Here's how the part is built. I have some questions about the finished solid (model axes, mm). Face numbers are marked on the shaded views. A direction names the side the tool comes from. Round coordinates to 2 decimals unless told otherwise and drop trailing zeros. Order: outer loops, then holes, each group sorted by start corner. A loop starts at its lowest first (then second) coordinate and runs counter-clockwise, first axis right, second up. Notation, with made-up numbers: (85, 45) - (110, 45) arc R18 ccw to (110, 66) - close; hole circle Ø6 at (88, -20). An arc over 180 degrees is marked (long way). One line per item, written item: value.
from build123d import *

# Parameters (mm, degrees)
SKETCH3_R                      = 5
BOTTOM_PLATE_DEPTH             = 5
SKETCH4_W                      = 5
SKETCH4_H                      = 343.002
VERTICAL_WALLS_DEPTH           = 400
MID_HORIZONTAL_PLATE_DEPTH     = 5
SKETCH7_W                      = 5
SKETCH7_H                      = 130.782
REST_OF_VERTICAL_EXTRUDE_DEPTH = 1560
SKETCH8_W                      = 280
SKETCH8_H                      = 130.782
TOP_PLATE_DEPTH                = 5
MOTOR_BOX_FILLETS_R            = 10
SKETCH10_W                     = 5
SKETCH10_H                     = 10
BOTTOM_PLATE_LIP_DEPTH         = 270


with BuildPart() as part:
    # Sketch3 → Bottom plate (new body)
    with BuildSketch(Plane.XZ.offset(985.61875)):
        Polygon((-140, 90.3875), (140, 90.3875), (140, -0.5375), (474.951, -0.5375), (474.951, -252.6145), (-140, -252.6145), align=None)
        with Locations(Location((88, -194.6125, 0), (0, 0, 270))):
            Circle(SKETCH3_R, mode=Mode.SUBTRACT)
        with Locations(Location((-93, -194.6125, 0), (0, 0, 270))):
            Circle(SKETCH3_R, mode=Mode.SUBTRACT)
        with Locations(Location((88, 7.3875, 0), (0, 0, 270))):
            Circle(SKETCH3_R, mode=Mode.SUBTRACT)
        with Locations(Location((-93, 7.3875, 0), (0, 0, 270))):
            Circle(SKETCH3_R, mode=Mode.SUBTRACT)
        with Locations(Location((-93, 78.3875, 0), (0, 0, 270))):
            Circle(SKETCH3_R, mode=Mode.SUBTRACT)
        with Locations(Location((88, 78.3875, 0), (0, 0, 270))):
            Circle(SKETCH3_R, mode=Mode.SUBTRACT)
    extrude(amount=BOTTOM_PLATE_DEPTH)

    # Sketch4 → Vertical walls (add)
    with BuildSketch(Plane(origin=(0, -985.61875, 0), x_dir=(1, 0, 0), z_dir=(0, 1, 0))):
        with Locations((-137.5, 81.1135)):
            Rectangle(SKETCH4_W, SKETCH4_H)
        Polygon((135, -90.3875), (135, 5.5375), (469.951, 5.5375), (469.951, 252.6145), (474.951, 252.6145), (474.951, 0.5375), (140, 0.5375), (140, -90.3875), align=None)
    extrude(amount=VERTICAL_WALLS_DEPTH)

    # Sketch6 → Mid horizontal plate (add)
    with BuildSketch(Plane(origin=(0, -585.61875, 0), x_dir=(1, 0, 0), z_dir=(0, 1, 0))):
        Polygon((135, -90.3875), (135, 35.3945), (-135, 35.3945), (-135, -90.3875), (-140, -90.3875), (-140, 252.6145), (-135, 252.6145), (135, 252.6145), (474.951, 252.6145), (474.951, 0.5375), (140, 0.5375), (140, -90.3875), align=None)
    extrude(amount=MID_HORIZONTAL_PLATE_DEPTH)

    # Sketch7 → Rest of vertical extrude (add)
    with BuildSketch(Plane(origin=(0, -580.61875, 0), x_dir=(1, 0, 0), z_dir=(0, 1, 0))):
        with Locations((137.5, -24.9965)):
            Rectangle(SKETCH7_W, SKETCH7_H)
        with Locations((-137.5, -24.9965)):
            Rectangle(SKETCH7_W, SKETCH7_H)
    extrude(amount=REST_OF_VERTICAL_EXTRUDE_DEPTH)

    # Sketch8 → Top plate (add)
    with BuildSketch(Plane(origin=(0, 979.38125, 0), x_dir=(1, 0, 0), z_dir=(0, 1, 0))):
        with Locations((0, -24.9965)):
            Rectangle(SKETCH8_W, SKETCH8_H)
    extrude(amount=TOP_PLATE_DEPTH)

    # Motor box fillets
    motor_box_fillets_edges = [part.edges().sort_by_distance(p)[0] for p in [
        (140, -580.61875, -20.466),
        (140, -785.61875, -0.5375),
        (474.951, -785.61875, -0.5375),
        (307.4755, -580.61875, -0.5375),
        (474.951, -580.61875, -126.576),
    ]]
    fillet(motor_box_fillets_edges, radius=MOTOR_BOX_FILLETS_R)

    # Sketch10 → Bottom plate lip (add)
    with BuildSketch(Plane.ZY.offset(-135)):
        with Locations((-32.8945, -580.61875)):
            Rectangle(SKETCH10_W, SKETCH10_H)
    extrude(amount=BOTTOM_PLATE_LIP_DEPTH)


solid = part.part
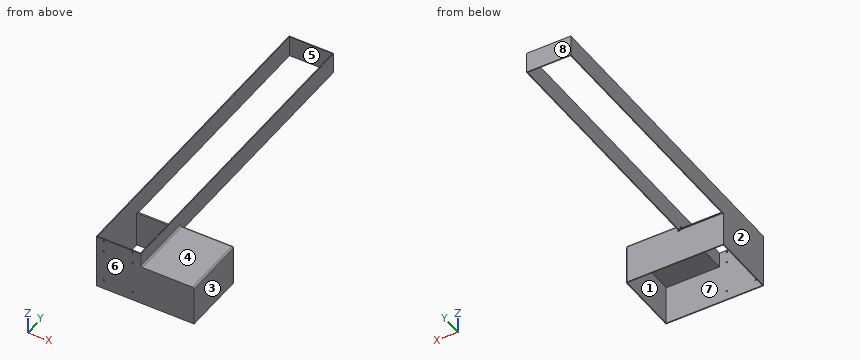
Q1. If we section it at C-C, the plane x = -16.5: Please give me the cut outline in (y, z), then the cut area to 3 significant figures.
Results list:
outline: (-990.62, -252.61) - (-985.62, -252.61) - (-985.62, 90.39) - (-990.62, 90.39) - close; (-585.62, -252.61) - (-580.62, -252.61) - (-580.62, -35.39) - (-575.62, -35.39) - (-575.62, -30.39) - (-585.62, -30.39) - close; (979.38, -40.39) - (984.38, -40.39) - (984.38, 90.39) - (979.38, 90.39) - close
area: 3,510 mm²
Q2. If we section it at B-B, the plane y = 445: Please give me the cut outline in (x, z).
Results list:
outline: (-140, -40.39) - (-135, -40.39) - (-135, 90.39) - (-140, 90.39) - close; (135, -40.39) - (140, -40.39) - (140, 90.39) - (135, 90.39) - close
Q3. Will these pins go through, and if not, where does the flat tip stop? pin 1 (16 mm diameter, centred on x = 88, z = 78.39, fed in from -Y); pin 2 (4 mm diameter, centred on y = -396, z = 37.5, fed in from +X); pin 3 (3 mm diameter, centred on x = 60, y = -582, fed in from +Z); pin 4 (8 mm diameter, centred on x = 88, z = -194.61, fed in from +Y).
Results list:
pin 1: y = -990.62
pin 2: x = 140
pin 3: z = -30.39
pin 4: y = -580.62
Q4. If we section it at D-D, the plane x = 318: Please give me the cut outline in (y, z).
Results list:
outline: (-990.62, -252.61) - (-985.62, -252.61) - (-985.62, -5.54) - (-585.62, -5.54) - (-585.62, -252.61) - (-580.62, -252.61) - (-580.62, -10.54) arc R10 ccw to (-590.62, -0.54) - (-990.62, -0.54) - close
Q5. We'd pull the mould along Y, two halves only. Please class the marked faces 6, 7 and 8: released by +Y, released by -Y, zero draft, split by the parting line, or undercut.
Results list:
face 6: released by -Y
face 7: undercut
face 8: released by +Y
Q6. Which directions (+Z, -Z, +X, -X, +Y, -Y) give clear straight access to the entire face, cutting with the end or side of a thin tool? Please do the marked faces 1, 2, 3, 4 and 5.
Results list:
face 1: -Z
face 2: +Z, -Z, -X, +Y, -Y
face 3: +Z, -Z, +X, +Y, -Y
face 4: +Z, +X, +Y, -Y
face 5: +Z, -Z
Q7. If I drill on line 1 along Y through (x, z) = (354, -35.5); line 2 along X through (y, z) = (112.5, -35); line 3 along X through (y, z) = (-862, -111), over which ranges is the centre line in solid material (lowest first)?
Results list:
line 1: -990.62 to -985.62, -585.62 to -580.62
line 2: -140 to -135, 135 to 140
line 3: -140 to -135, 469.95 to 474.95
Q8. If we section it at A-A, the plane z = -219: Please give me the cut outline in (x, y), then the cut area to 3 significant figures.
Results list:
outline: (-140, -990.62) - (474.95, -990.62) - (474.95, -590.62) arc R10 ccw to (464.95, -580.62) - (-140, -580.62) - close; hole (-135, -985.62) - (469.95, -985.62) - (469.95, -585.62) - (-135, -585.62) - close
area: 10,100 mm²
